Geometry: final body of the model. Coordinates: model frame, mm. Give positions to 0.01 mm unless a question says otherwise; leave off trailing zeros. Write each loop counter-clockwise with the first axis right and the second up, starting at its lowest first coordinate (ties: lowest second). Pieces come first, ordered by that corner, then holes. Notation, with made-up numbers: M 24.25,55.25 L 45.25,55.25 A33 ccw 45.25,86.25 Z; hole C -34.75,-7.75 d7. An arc over 180 degrees is marked long. One line per question, with ' | ' between items.
from build123d import *

# Parameters (mm, degrees)
SKETCH1_W                  = 177.8
SKETCH1_H                  = 63.5
SKETCH1_R                  = 6.35
SKETCH1_R_2                = 14.2875
BOSS_EXTRUDE2_DEPTH        = 6.35
F_9_0_196_DIAMETER_HOLE1_D = 4.9784


with BuildPart() as part:
    # Sketch1 → Boss-Extrude2 (new body)
    with BuildSketch(Plane.XY):
        with Locations((0, 49.5808)):
            Rectangle(SKETCH1_W, SKETCH1_H)
        with Locations((-41.221968309, 29.688201844)):
            Circle(SKETCH1_R, mode=Mode.SUBTRACT)
        with Locations((0, 49.5808)):
            Circle(SKETCH1_R_2, mode=Mode.SUBTRACT)
        with Locations((41.221968309, 29.688201844)):
            Circle(SKETCH1_R, mode=Mode.SUBTRACT)
    extrude(amount=BOSS_EXTRUDE2_DEPTH)

    # #9 (0.196) Diameter Hole1 (through all)
    with Locations(Plane(origin=(0, 0, 0), x_dir=(-1, 0, 0), z_dir=(0, 0, -1))):
        with Locations((-82.55, 74.9808), (-82.55, 24.1808), (82.55, 24.1808), (82.55, 74.9808)):
            Hole(F_9_0_196_DIAMETER_HOLE1_D / 2)


solid = part.part
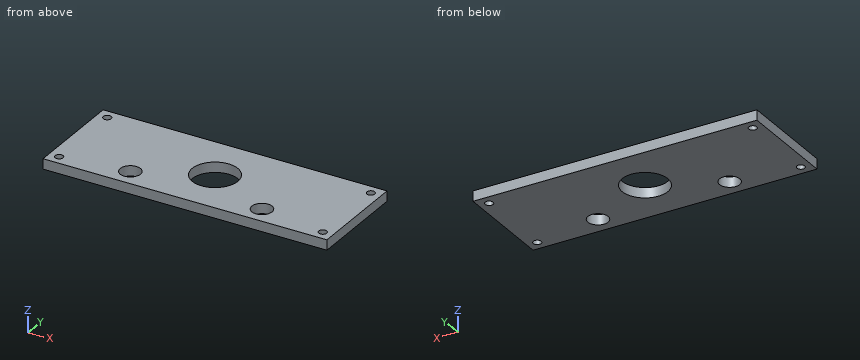
(1) First-contact query: P1, Ø6.5, axis at x = 82.55, y = 24.18, coming from the +Z side; P2, Ø10, axis at x = -41.22, y = 29.69, coming from the +Z side. Flat tips, straight axial feed; report the tip coordinate or a pass-through.
Working result:
P1: stops at z = 6.35 | P2: passes through
(2) Cut plane C-C, the plane y = 59.5. Return loops of the section in (x, z).
Working result:
outline: M -88.9,0 L -10.28,0 L -10.28,6.35 L -88.9,6.35 Z; M 10.28,0 L 88.9,0 L 88.9,6.35 L 10.28,6.35 Z
(3) Cut plane B-B, the plane x = 0. Return loops of the section in (y, z).
Working result:
outline: M 17.83,0 L 35.29,0 L 35.29,6.35 L 17.83,6.35 Z; M 63.87,0 L 81.33,0 L 81.33,6.35 L 63.87,6.35 Z
(4) Cut plane A-A, the plane x = 82.55. Return loops of the section in (y, z), then the cut area to 3 significant figures.
Working result:
outline: M 17.83,0 L 21.69,0 L 21.69,6.35 L 17.83,6.35 Z; M 26.67,0 L 72.49,0 L 72.49,6.35 L 26.67,6.35 Z; M 77.47,0 L 81.33,0 L 81.33,6.35 L 77.47,6.35 Z | area: 340 mm^2
(5) Material intervals for L1, parallel to Y at x = 82.55, z = 5.25; L2, parallel to Y at x = -0.5, z = 1.25; L3, parallel to X at y = 75, z = 2, sorted ascending. Write a range as [from, to].
Working result:
L1: y = [17.83, 21.69], [26.67, 72.49], [77.47, 81.33] | L2: y = [17.83, 35.3], [63.86, 81.33] | L3: x = [-88.9, -85.04], [-80.06, 80.06], [85.04, 88.9]
(6) Cut plane D-D, the plane z = 2.5. Count the separate pieces of the cut face and the enclosed holes in it, then the cut area to 3 significant figures.
Working result:
separate pieces: 1 | enclosed holes: 7 | area: 10,300 mm^2
